```python
from build123d import *

# Parameters (mm, degrees)
F0_W         = 54
F0_H         = 54
F1_DEPTH     = 2
F2_R         = 3
F3_T1_DEPTH  = 48
F3_T3_DEPTH  = 48
F3_T6_ANGLE  = 90
F3_T8_ANGLE  = 90
F3_T10_ANGLE = 90
F3_T12_ANGLE = 90
F4_W         = 50.1
F4_H         = 50.1
F4_W_2       = 48
F4_H_2       = 48
F5_DEPTH     = 2
F6_R         = 2.5
F6_R_2       = 1.4
F7_DEPTH     = 3
F8_R         = 2
F9_R         = 2.6
F9_R_2       = 1.5
F10_DEPTH    = 3
F11_R        = 1.5
F12_DEPTH    = 25


# Not quite as in the source:
# - a fillet or chamfer that OpenCascade refuses, or shapes differently, is made with other operations: its cross-section is extruded or revolved along the edge and cut away or added


with BuildPart() as f1:
    # F0 (on Top) → F1 (new body)
    with BuildSketch(Plane.XY):
        Rectangle(F0_W, F0_H)
    extrude(amount=F1_DEPTH)

    # F2
    f2_edges = [f1.edges().sort_by_distance(p)[0] for p in [
        (-27, -27, 1),
        (-27, 27, 1),
        (27, 27, 1),
        (27, -27, 1),
    ]]
    fillet(f2_edges, radius=F2_R)

    # F3: fillet of radius 3 on 8 edges, made by hand

    # F3_s2 → F3_t1 (cut)
    with BuildSketch(Plane.YZ.offset(-24)):
        with BuildLine():
            ThreePointArc((27, 2), (25.9036236828, 0.5505102572), (24.1715728753, 0))
            Line((24.1715728753, 0), (27, 0))
            Line((27, 0), (27, 2))
        make_face()
        with BuildLine():
            ThreePointArc((-24.1715728753, 0), (-25.9036236828, 0.5505102572), (-27, 2))
            Line((-27, 2), (-27, 0))
            Line((-27, 0), (-24.1715728753, 0))
        make_face()
    extrude(amount=F3_T1_DEPTH, mode=Mode.SUBTRACT)

    # F3_s4 → F3_t3 (cut)
    with BuildSketch(Plane.XZ.offset(-24)):
        with BuildLine():
            ThreePointArc((24.1715728753, 0), (25.9036236828, 0.5505102572), (27, 2))
            Line((27, 2), (27, 0))
            Line((27, 0), (24.1715728753, 0))
        make_face()
        with BuildLine():
            ThreePointArc((-24.1715728753, 0), (-25.9036236828, 0.5505102572), (-27, 2))
            Line((-27, 2), (-27, 0))
            Line((-27, 0), (-24.1715728753, 0))
        make_face()
    extrude(amount=F3_T3_DEPTH, mode=Mode.SUBTRACT)

    # F3_s5 → F3_t6 (revolve, cut)
    with BuildSketch(Plane.YZ.offset(24)):
        with BuildLine():
            ThreePointArc((24.1715728753, 0), (25.9036236828, 0.5505102572), (27, 2))
            Line((27, 2), (27, 0))
            Line((27, 0), (24.1715728753, 0))
        make_face()
    revolve(axis=Axis((24, 24, 0), (0, 0, -1)), revolution_arc=F3_T6_ANGLE, mode=Mode.SUBTRACT)

    # F3_s7 → F3_t8 (revolve, cut)
    with BuildSketch(Plane.YZ.offset(-24)):
        with BuildLine():
            ThreePointArc((24.1715728753, 0), (25.9036236828, 0.5505102572), (27, 2))
            Line((27, 2), (27, 0))
            Line((27, 0), (24.1715728753, 0))
        make_face()
    revolve(axis=Axis((-24, 24, 0), (0, 0, 1)), revolution_arc=F3_T8_ANGLE, mode=Mode.SUBTRACT)

    # F3_s9 → F3_t10 (revolve, cut)
    with BuildSketch(Plane.YZ.offset(24)):
        with BuildLine():
            ThreePointArc((-24.1715728753, 0), (-25.9036236828, 0.5505102572), (-27, 2))
            Line((-27, 2), (-27, 0))
            Line((-27, 0), (-24.1715728753, 0))
        make_face()
    revolve(axis=Axis((24, -24, 0), (0, 0, 1)), revolution_arc=F3_T10_ANGLE, mode=Mode.SUBTRACT)

    # F3_s11 → F3_t12 (revolve, cut)
    with BuildSketch(Plane.XZ.offset(24)):
        with BuildLine():
            ThreePointArc((-24.1715728753, 0), (-25.9036236828, 0.5505102572), (-27, 2))
            Line((-27, 2), (-27, 0))
            Line((-27, 0), (-24.1715728753, 0))
        make_face()
    revolve(axis=Axis((-24, -24, 0), (0, 0, 1)), revolution_arc=F3_T12_ANGLE, mode=Mode.SUBTRACT)

    # F4 (on face) → F5 (join)
    with BuildSketch(Plane.XY.offset(2)):
        Rectangle(F4_W, F4_H)
        Rectangle(F4_W_2, F4_H_2, mode=Mode.SUBTRACT)
    extrude(amount=F5_DEPTH)

    # F6 (on face) → F7 (join)
    with BuildSketch(Plane.XY.offset(2)):
        with Locations((-22.5, 22.5)):
            Circle(F6_R)
        with Locations((-22.5, 22.5)):
            Circle(F6_R_2, mode=Mode.SUBTRACT)
        with Locations((22.5, 22.5)):
            Circle(F6_R)
        with Locations((22.5, 22.5)):
            Circle(F6_R_2, mode=Mode.SUBTRACT)
        with Locations((22.5, -22.5)):
            Circle(F6_R)
        with Locations((22.5, -22.5)):
            Circle(F6_R_2, mode=Mode.SUBTRACT)
        with Locations((-22.5, -22.5)):
            Circle(F6_R)
        with Locations((-22.5, -22.5)):
            Circle(F6_R_2, mode=Mode.SUBTRACT)
    extrude(amount=F7_DEPTH)

    # F8
    f8_edges = [f1.edges().sort_by_distance(p)[0] for p in [
        (-25.05, -25.05, 3),
        (25.05, -25.05, 3),
        (25.05, 25.05, 3),
        (-25.05, 25.05, 3),
    ]]
    fillet(f8_edges, radius=F8_R)

    # F9 (on face) → F10 (join)
    with BuildSketch(Plane.XY.offset(2)):
        with Locations((22.3, 0.8)):
            Circle(F9_R)
        with Locations((22.3, 0.8)):
            Circle(F9_R_2, mode=Mode.SUBTRACT)
        with Locations((22.3, -6.6)):
            Circle(F9_R)
        with Locations((22.3, -6.6)):
            Circle(F9_R_2, mode=Mode.SUBTRACT)
    extrude(amount=F10_DEPTH)

    # F11 (on face) → F12 (cut)
    with BuildSketch(Plane.XY.offset(2)):
        with Locations((22.3, 0.8)):
            Circle(F11_R)
        with Locations((22.3, -6.6)):
            Circle(F11_R)
    extrude(amount=-F12_DEPTH, mode=Mode.SUBTRACT)


solid = f1.part
```
Could you check a few things on this model? Use its own coordinates, in mm. A direction names the side the tool comes from. Coordinates: 2 decimals unless noted, no trailing zeros. Loops run counter-clockwise (first coordinate to the right, second up) from the corner with the lowest first, then second, coordinate; pieces in that order, holes last.
1) Imagine slicing it at D-D (z = 1.3). State how many separate pieces and enclosed holes the cut face has, and give its area (3 significant figures).
Reported:
separate pieces: 1
enclosed holes: 2
area: 2,820 mm2
2) Will these pins go through, and if not, where does the flat tip stop? pin 1 Ø2 at (x, y) = (22.5, 22.5) entering from +Z; pin 2 Ø1.8 at (x, y) = (22.3, -6.6) entering from +Z; pin 3 Ø0.6 at (x, z) = (6, 3) entering from +Y; pin 4 Ø2 at (x, z) = (-7, 2.5) entering from -Y.
Reported:
pin 1: stops at z = 2
pin 2: passes through
pin 3: stops at y = 25.05
pin 4: stops at y = -27
3) Thinking about a two-plate mould opening in Y: for faces 4 (the face through (0, 25.05, 3)), 5 (the face through (23.15, 21.26, 3.48)), 6 (the face through (-0.336, -25.882, 0.536)), which applies, released by +Y, released by -Y, zero draft, split by the parting line, or undercut?
Reported:
face 4: released by +Y
face 5: undercut
face 6: released by -Y
4) Imagine slicing it at A-A (y = 0.8). List the corners of the cut face in (x, z) for me.
Reported:
outline: (-27, 2) arc R3 ccw to (-24.17, 0) - (20.8, 0) - (20.8, 5) - (19.7, 5) - (19.7, 2) - (-24, 2) - (-24, 4) - (-25.05, 4) - (-25.05, 2) - close; (23.8, 0) - (24.17, 0) arc R3 ccw to (27, 2) - (25.05, 2) - (25.05, 4) - (24.9, 4) - (24.9, 5) - (23.8, 5) - close
5) Please list where these lines run through material, in increasing order: line 1 along Y through (x, z) = (-22.5, 3.2); line 2 along Y through (x, z) = (18.5, 2.85); line 3 along X through (y, z) = (23, 3.15).
Reported:
line 1: y = -25.05 to -23.9, -21.1 to -20, 20 to 21.1, 23.9 to 25.05
line 2: y = -25.05 to -24, 24 to 25.05
line 3: x = -25.05 to -23.81, -21.19 to -20.05, 20.05 to 21.19, 23.81 to 25.05
6) Imagine slicing it at B-B (x = -16). List the corners of the cut face in (y, z) for me.
Reported:
outline: (-27, 2) arc R3 ccw to (-24.17, 0) - (24.17, 0) arc R3 ccw to (27, 2) - (25.05, 2) - (25.05, 4) - (24, 4) - (24, 2) - (-24, 2) - (-24, 4) - (-25.05, 4) - (-25.05, 2) - close
7) Which directions (+Z, -Z, +X, -X, +Y, -Y) give clear straight access to the entire face, cutting with the end or side of a thin tool? Please do faces 1 (the face through (25.05, 0, 3)), 2 (the face through (0, -25.05, 3)), 3 (the face through (0, -26, 2)).
Reported:
face 1: +Z, +X, +Y, -Y
face 2: +Z, +X, -X, -Y
face 3: +Z
